The listing builds one solid part. Answer for the finished solid, in the listing's coordinates (mm). Face numbers are marked on the shaded views. A direction names the side the tool comes from. Round coordinates to 2 decimals unless told otherwise and drop trailing zeros. Order: outer loops, then holes, each group sorted by start corner. A loop starts at its lowest first (then second) coordinate and runs counter-clockwise, first axis right, second up. Notation, with made-up numbers: (3.5, -11) - (47.5, -11) arc R25 ccw to (47.5, 15) - close; hole circle Ø7 at (67, 12.25). An arc over 180 degrees is marked (long way). Use CSV: the item, a comma, the result in double quotes. Start each with the question number.
Item 1: Flat-ended cylindrical pins translate along their axes: P1, Ø13, axis at y = 1.5, z = 22, coming from the +X side; P2, Ø1.5, axis at x = 10, z = 13.5, coming from the +Y side; P3, Ø8, axis at x = 2, z = 18, coming from the +Y side; P4, Ø17.5, axis at x = -2.5, z = 19.5, coming from the -Y side. Find the tip coordinate at first contact, or state that the pin passes through.
Item 2: For the marked faces 1, 2, 3 and 4, determine the directions among +Z, -Z, +X, -X, +Y, -Y from which every point of the face is accessible in a straight line to the end or side of a thin tool.
Item 3: Straight lines are drawn through the part: line 1 along Z through (x, y) = (17, 11); line 2 along X through (y, z) = (-8, 3.5). For each, find the intervals that lie inside material, in ascending order. Write a range as [from, to].
Item 4: Find section A-A, the plane x = -6.5. Give the vertices of the cut face in (y, z).
Item 5: Find section C-C, the plane x = -15. Give the vertices of the cut face in (y, z), plus the area to 3 significant figures.
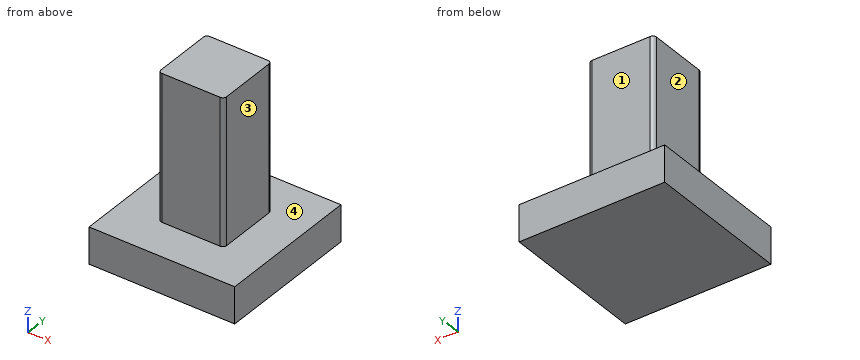
Autodesk Inventor part; units mm, degrees
ref_plane "YZ Plane" through (0, 0, 0) normal (1, 0, 0) x (0, 1, 0)
ref_plane "XZ Plane" through (0, 0, 0) normal (0, 1, 0) x (-1, 0, 0)
ref_plane "XY Plane" through (0, 0, 0) normal (0, 0, 1) x (1, 0, 0)
sketch "Náčrt1" plane through (0, 0, 0) normal (0, 0, 1) x (1, 0, 0)
  line L0 (-9, -9) -> (9, -9)
  line L1 (9, -9) -> (9, 9)
  line L2 (9, 9) -> (-9, 9)
  line L3 (-9, 9) -> (-9, -9)
  line L4 (-9, -9) -> (9, 9) construction
  line L5 (9, -9) -> (-9, 9) construction
  line L6 (20, -20) -> (-20, -20)
  line L7 (-20, -20) -> (-20, 20)
  line L8 (-20, 20) -> (20, 20)
  line L9 (20, 20) -> (20, -20)
  line L10 (20, -20) -> (-20, 20) construction
  line L11 (-20, -20) -> (20, 20) construction
  point P0 (0, 0)
  dimension "d0" = 18
  dimension "d1" = 18
  dimension "d2" = 40
  dimension "d3" = 40
extrude "Vysunutí1" add sketch "Náčrt1" along normal blind 40 contours L3 L2 L1 L0
extrude "Vysunutí2" add sketch "Náčrt1" against normal blind 10 contours L3 L2 L1 L0 | L6 L7 L8 L9
fillet "Zaoblení1" radius 1 4 edges at (9, 9, 20) (9, -9, 20) (-9, -9, 20) (-9, 9, 20)
properties part number "motor držák"
Worked out:
1,P1,"stops at x = 9"
1,P2,"passes through"
1,P3,"stops at y = 9"
1,P4,"stops at y = -9"
2,face 1,"+Z, +X, -X, +Y"
2,face 2,"+Z, -X, +Y, -Y"
2,face 3,"+Z, +X, +Y, -Y"
2,face 4,"+Z"
3,line 1,"z = [-10, 0]"
3,line 2,"x = [-9, 9]"
4,outline,"(-20, -10) - (20, -10) - (20, 0) - (9, 0) - (9, 40) - (-9, 40) - (-9, 0) - (-20, 0) - close"
5,outline,"(-20, -10) - (20, -10) - (20, 0) - (-20, 0) - close"
5,area,"400 mm²"
